Could you check a few things on this drawing? It's one solid part, dimensions in mm from its lowest x, y, z. Round coordinates to 2 decimals unless told otherwise and drop trailing zeros. Write each loop counter-clockwise with the first axis right and the second up, starting at its lowest first coordinate (ties: lowest second). Pieces come first, ordered by that corner, then holes. Notation, with made-up numbers: (29, -3.75) - (55, -3.75) arc R14 ccw to (55, 5.25) - close; hole circle Ø10 at (38, 24.5). An arc over 180 degrees is marked (long way). Use one line per item in the form item = value. Start each with the question number.
1. Will these pins go through, and if not, where does the flat tip stop? pin 1 (1.5 mm diameter, centred on y = 20, z = 100.5, fed in from +X); pin 2 (3 mm diameter, centred on y = 27, z = 50, fed in from +X).
2. If I drill on line 1 along X through (y, z) = (29, 131.5); line 2 along X through (y, z) = (3, 126.5) (1 decimal); line 3 along Y through (x, z) = (54, 102.5), over which ranges is the centre line in solid material (lowest first)?
3. I want a section at C-C, the plane x = 63. List the corners of the cut face in (y, z) for me.
4. I want a section at A-A, the plane z = 41. List the corners of the cut face in (x, y) for me.
5. I want a section at B-B, the plane y = 16.5. List the corners of the cut face in (x, z) for me.
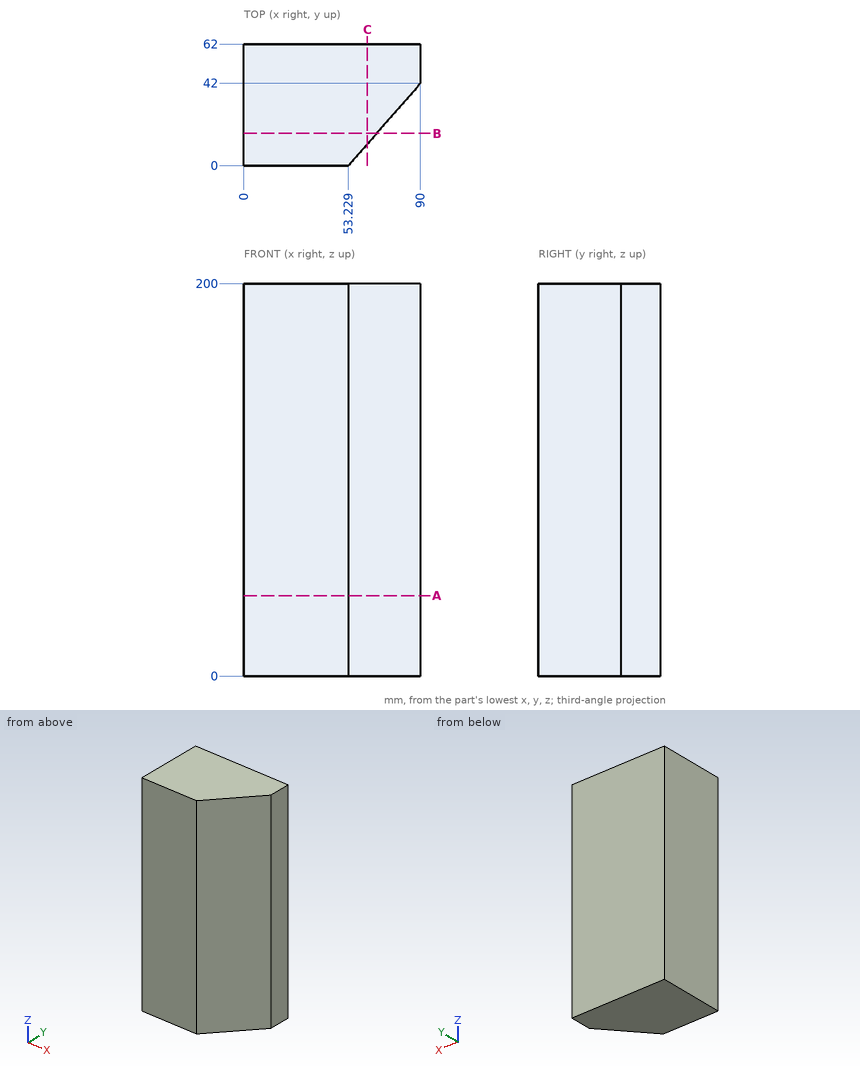
Model answer:
q1.pin_1 = 71.4
q1.pin_2 = 78.18
q2.line_1 = 0 to 78.62
q2.line_2 = 0 to 55.9
q2.line_3 = 0.88 to 62
q3.outline = (11.16, 0) - (62, 0) - (62, 200) - (11.16, 200) - close
q4.outline = (0, 0) - (53.23, 0) - (90, 42) - (90, 62) - (0, 62) - close
q5.outline = (0, 0) - (67.67, 0) - (67.67, 200) - (0, 200) - close
